Design review of the part shown in the three views and the two pictorial views. Dimensions are in mm from the part's minimum x, y and z. Coordinates: 2 decimals unless noted, no trailing zeros. Write each loop counter-clockwise with the first axis right and the second up, starting at its lowest first coordinate (ties: lowest second). Pieces come first, ordered by that corner, then holes. Notation, with made-up numbers: (19, 21.5) - (47, 21.5) arc R3 cw to (47, 26.5) - close; hole circle Ø10 at (59.5, 76.25). An arc over 180 degrees is marked (long way). Write each question's results on one line, items separated by ' | '.
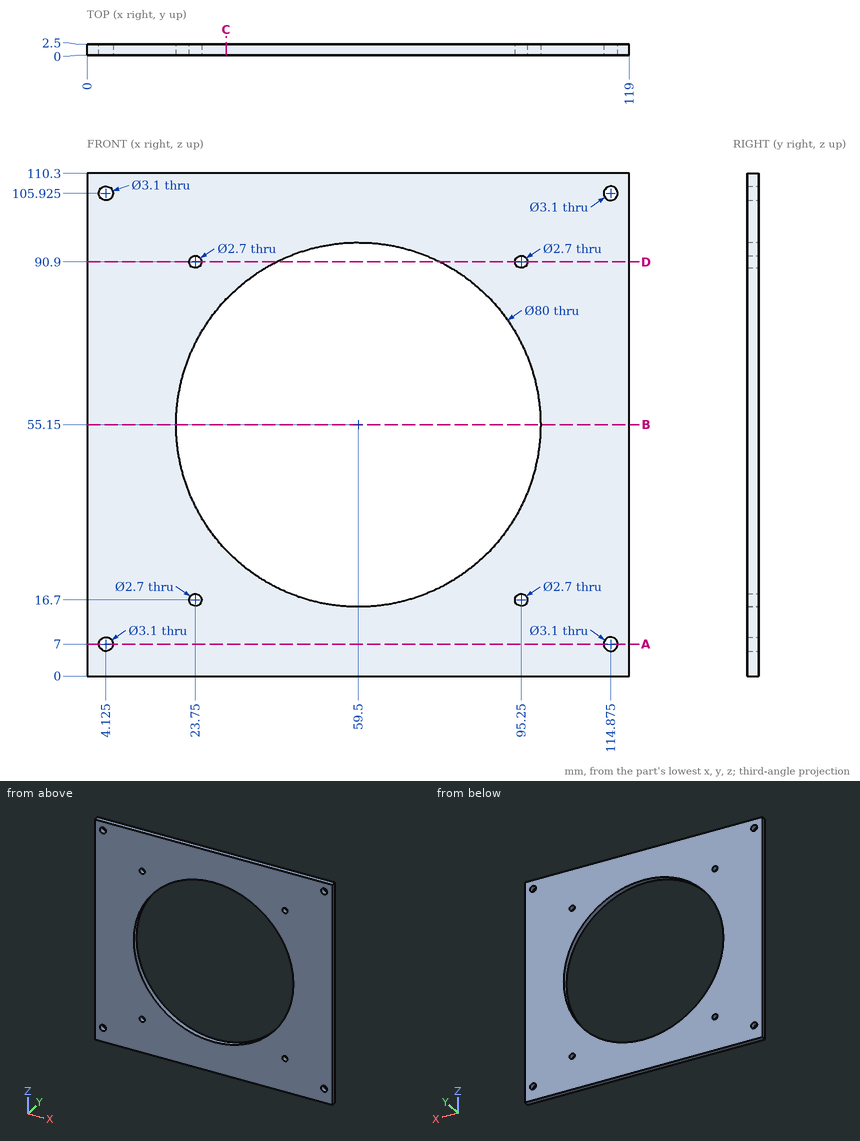
Q1. Take a section at B-B on z = 55.15. State the section outline as (x, y) points, plus the area to 3 significant figures.
Results found:
outline: (0, 0) - (19.5, 0) - (19.5, 2.5) - (0, 2.5) - close; (99.5, 0) - (119, 0) - (119, 2.5) - (99.5, 2.5) - close | area: 97.5 mm2
Q2. Take a section at C-C on x = 30.5. State the section outline as (y, z) points.
Results found:
outline: (0, 0) - (2.5, 0) - (2.5, 27.6) - (0, 27.6) - close; (0, 82.7) - (2.5, 82.7) - (2.5, 110.3) - (0, 110.3) - close
Q3. For pin 1 (4.5 mm diameter, centred on x = 95.25, z = 16.7, fed in from +Y), flat-tipped, find the tip position at first contact; note if it passes through.
Results found:
pin 1: y = 2.5
Q4. Take a section at D-D on z = 90.9. State the section outline as (x, y) points, plus the area to 3 significant figures.
Results found:
outline: (0, 0) - (22.4, 0) - (22.4, 2.5) - (0, 2.5) - close; (25.1, 0) - (41.56, 0) - (41.56, 2.5) - (25.1, 2.5) - close; (77.44, 0) - (93.9, 0) - (93.9, 2.5) - (77.44, 2.5) - close; (96.6, 0) - (119, 0) - (119, 2.5) - (96.6, 2.5) - close | area: 194 mm2
Q5. Take a section at A-A on z = 7. State the section outline as (x, y) points (3 decimals).
Results found:
outline: (0, 0) - (2.575, 0) - (2.575, 2.5) - (0, 2.5) - close; (5.675, 0) - (113.325, 0) - (113.325, 2.5) - (5.675, 2.5) - close; (116.425, 0) - (119, 0) - (119, 2.5) - (116.425, 2.5) - close
Q6. Wall thickness on line 1 along Z through (x, y) = (59.5, 1.65); line 2 along X through (y, z) = (1.35, 90.9); line 3 along X through (y, z) = (1.05, 91): over which ranges is each line inside the solid? List them lowest first. Write a range as from..to.
Results found:
line 1: 0..15.15, 95.15..110.3 | line 2: 0..22.4, 25.1..41.56, 77.44..93.9, 96.6..119 | line 3: 0..22.4, 25.1..41.76, 77.24..93.9, 96.6..119
